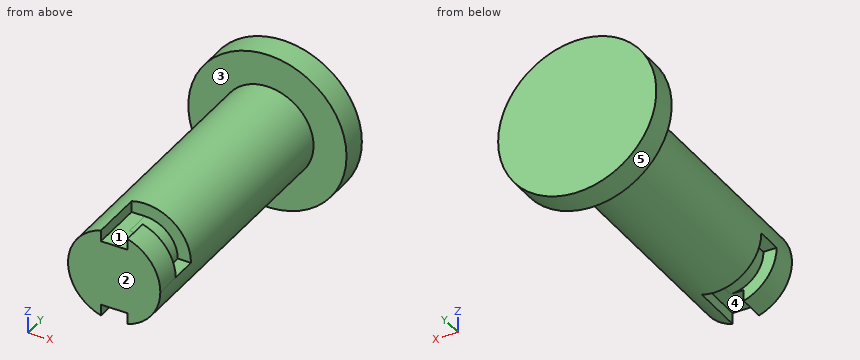
from build123d import *

# Parameters (mm, degrees)
SKETCH1_R           = 3.5
BOSS_EXTRUDE1_DEPTH = 20
SKETCH2_R           = 6
BOSS_EXTRUDE2_DEPTH = 2
CUT_EXTRUDE1_DEPTH  = 4
SKETCH6_W           = 1
SKETCH6_H           = 2
CUT_REVOLVE1_ANGLE  = 90


with BuildPart() as part:
    # Sketch1 → Boss-Extrude1 (new body)
    with BuildSketch(Plane(origin=(0, 0, 0), x_dir=(1, 0, 0), z_dir=(0, 1, 0))):
        Circle(SKETCH1_R)
    extrude(amount=BOSS_EXTRUDE1_DEPTH)

    # Sketch2 → Boss-Extrude2 (add)
    with BuildSketch(Plane(origin=(0, 20, 0), x_dir=(1, 0, 0), z_dir=(0, 1, 0))):
        Circle(SKETCH2_R)
    extrude(amount=BOSS_EXTRUDE2_DEPTH)

    # Sketch3 → Cut-Extrude1 (cut)
    with BuildSketch(Plane.XZ):
        Polygon((0, 3.5), (-1, 3.5), (-1, 2.5), (1, 2.5), (1, 3.5), align=None)
        Polygon((-1, -3.5), (-1, -2.5), (1, -2.5), (1, -3.5), (0, -3.5), align=None)
    extrude(amount=-CUT_EXTRUDE1_DEPTH, mode=Mode.SUBTRACT)

    # Sketch6 → Cut-Revolve1 (revolve, cut)
    with BuildSketch(Plane(origin=(0, 0, 0), x_dir=(0, 0, -1), z_dir=(1, 0, 0))):
        with Locations((3, 3)):
            Rectangle(SKETCH6_W, SKETCH6_H)
        with Locations((-3, 3)):
            Rectangle(SKETCH6_W, SKETCH6_H)
    revolve(axis=Axis((0, 0, 0), (0, 1, 0)), revolution_arc=CUT_REVOLVE1_ANGLE, mode=Mode.SUBTRACT)


solid = part.part
Geometry: final body of the model. Coordinates: model frame, mm. Face numbers are marked on the shaded views. A direction names the side the tool comes from. Coordinates: 2 decimals unless noted, no trailing zeros. Order: outer loops, then holes, each group sorted by start corner. A loop starts at its lowest first (then second) coordinate and runs counter-clockwise, first axis right, second up.
1) Draft query along X for the marked faces 3, 4 and 5. Return one class per face: released by +X, released by -X, zero draft, split by the parting line, or undercut.
Result sheet:
face 3: zero draft
face 4: undercut
face 5: split by the parting line
2) Set-up query: the marked faces 1 and 2. Return all of +Z, -Z, +X, -X, +Y, -Y with unobstructed straight access to the full face (end or side cutting, diameter ignored); none if empty.
Result sheet:
face 1: +Z, -Y
face 2: +Z, -Z, +X, -X, -Y
3) First-contact query: P1, Ø2, axis at x = 0.5, y = 1.5, coming from the +Z side; P2, Ø0.9, axis at y = 1, z = -3, coming from the -X side; P3, Ø4, axis at y = 5, z = 0.5, coming from the +X side. Flat tips, straight axial feed; report the tip coordinate or a pass-through.
Result sheet:
P1: stops at z = 3.35
P2: stops at x = -2.4
P3: stops at x = 3.5
4) Section A-A (z = -2.75). Return loops of the section in (x, y), then the cut area to 3 significant figures.
Result sheet:
outline: (-5.33, 20) - (-2.17, 20) - (-2.17, 4) - (1, 4) - (1, 0) - (2.17, 0) - (2.17, 20) - (5.33, 20) - (5.33, 22) - (-5.33, 22) - close; (-2.17, 0) - (-1, 0) - (-1, 2) - (-2.17, 2) - close
area: 97.6 mm2
5) Ray query, probe 1 along Y at (x, z) = (-3.75, 0.75); probe 2 along X at (y, z) = (12.5, 1). Return the intervals inside material, ascending.
Result sheet:
probe 1: y = 20 to 22
probe 2: x = -3.35 to 3.35
6) Section B-B (x = 2.75). Return loops of the section in (y, z).
Result sheet:
outline: (0, -2.17) - (20, -2.17) - (20, -5.33) - (22, -5.33) - (22, 5.33) - (20, 5.33) - (20, 2.17) - (4, 2.17) - (4, 0) - (2, 0) - (2, 2.17) - (0, 2.17) - close
7) Section C-C (y = 16). Return loops of the section in (x, z).
Result sheet:
outline: circle Ø7 at (0, 0)
8) Section D-D (z = 2). Return loops of the section in (x, y).
Result sheet:
outline: (-5.66, 20) - (-2.87, 20) - (-2.87, 0) - (2.87, 0) - (2.87, 2) - (1.5, 2) - (1.5, 4) - (2.87, 4) - (2.87, 20) - (5.66, 20) - (5.66, 22) - (-5.66, 22) - close
